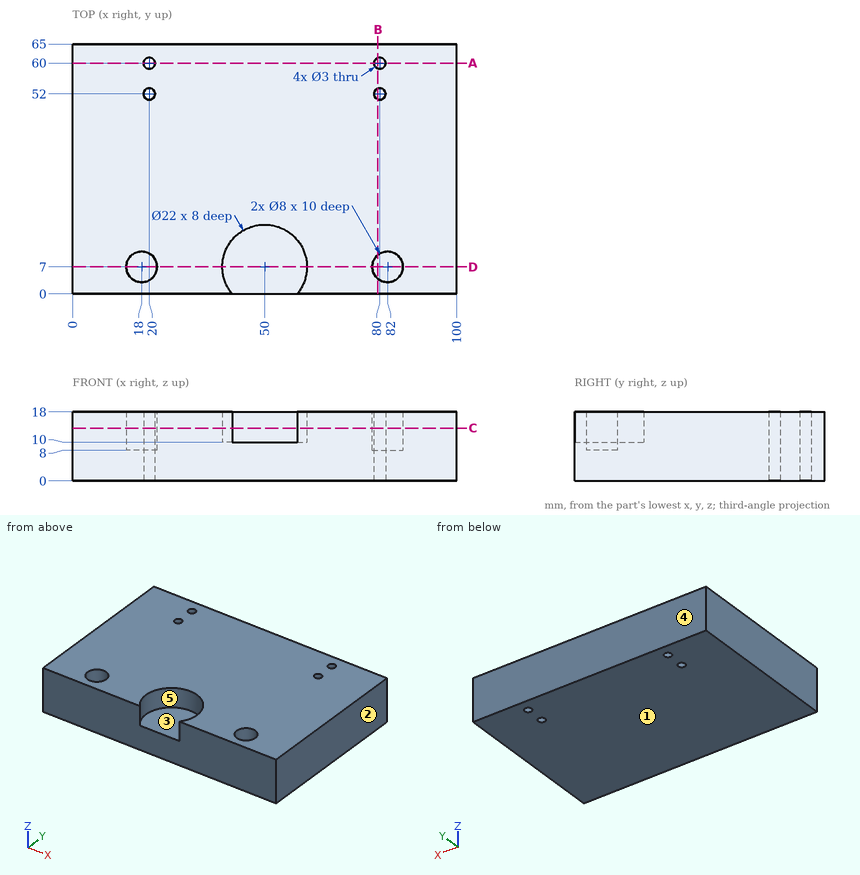
Part print with two shaded views. Sizes in mm from the minimum x, y, z corner. A direction names the side the tool comes from. Round coordinates to 2 decimals unless told otherwise and drop trailing zeros. Order: outer loops, then holes, each group sorted by start corner. A loop starts at its lowest first (then second) coordinate and runs counter-clockwise, first axis right, second up. Notation, with made-up numbers: (-33.5, 14.25) -> (1.5, 14.25) arc R16 cw to (1.5, 44.25) -> close; hole circle Ø2 at (8.25, 87). An arc over 180 degrees is marked (long way). Use one line per item in the form item = value.
Item 1: Drill centre lines: line 1 (Y direction, x = 20, z = 6.5); line 2 (Y direction, x = 82, z = 12.75); line 3 (X direction, y = 8, z = 13). Where is each one in solid material? Low to high.
Returned:
line_1 = 0 to 50.5, 53.5 to 58.5, 61.5 to 65
line_2 = 0 to 3, 11 to 65
line_3 = 0 to 14.13, 21.87 to 39.05, 60.95 to 78.13, 85.87 to 100
Item 2: Cut at B-B, the plane x = 79.5. Write the cut outline in (y, z), and give its area (3 significant figures).
Returned:
outline = (0, 0) -> (50.59, 0) -> (50.59, 18) -> (10.12, 18) -> (10.12, 8) -> (3.88, 8) -> (3.88, 18) -> (0, 18) -> close; (53.41, 0) -> (58.59, 0) -> (58.59, 18) -> (53.41, 18) -> close; (61.41, 0) -> (65, 0) -> (65, 18) -> (61.41, 18) -> close
area = 1,010 mm^2
Item 3: Cut at D-D, the plane y = 7. Write the cut outline in (x, z).
Returned:
outline = (0, 0) -> (100, 0) -> (100, 18) -> (86, 18) -> (86, 8) -> (78, 8) -> (78, 18) -> (61, 18) -> (61, 10) -> (39, 10) -> (39, 18) -> (22, 18) -> (22, 8) -> (14, 8) -> (14, 18) -> (0, 18) -> close
Item 4: Cut at A-A, the plane y = 60. Write the cut outline in (x, z), and give its area (3 significant figures).
Returned:
outline = (0, 0) -> (18.5, 0) -> (18.5, 18) -> (0, 18) -> close; (21.5, 0) -> (78.5, 0) -> (78.5, 18) -> (21.5, 18) -> close; (81.5, 0) -> (100, 0) -> (100, 18) -> (81.5, 18) -> close
area = 1,690 mm^2
Item 5: Tool access for the marked faces 4 and 5: list every direction of +Z, -Z, +X, -X, +Y, -Y with a clear straight run to the whole face (end or side of a thin tool).
Returned:
face_4 = +Z, -Z, +X, -X, +Y
face_5 = +Z
Item 6: Flat gauge pins, fed straight in: pin 1 Ø5.5 at (x, y) = (50.5, 8.5) entering from +Z; pin 2 Ø6.5 at (x, y) = (80.5, 6.5) entering from +Z; pin 3 Ø7 at (x, y) = (82, 7) entering from +Z. Where does each tip first touch, or does it go through?
Returned:
pin_1 = 10
pin_2 = 18
pin_3 = 8
Item 7: Pull direction X, two halves, no side cores. Call the marked faces 1, 2 and 3: released by +X, released by -X, zero draft, split by the parting line, or undercut.
Returned:
face_1 = zero draft
face_2 = released by +X
face_3 = undercut
Item 8: Cut at C-C, the plane z = 13.75. Write the cut outline in (x, y), and give its area (3 significant figures).
Returned:
outline = (0, 0) -> (41.51, 0) arc R11 cw (long way) to (58.49, 0) -> (100, 0) -> (100, 65) -> (0, 65) -> close; hole circle Ø8 at (18, 7); hole circle Ø3 at (20, 52); hole circle Ø3 at (20, 60); hole circle Ø8 at (82, 7); hole circle Ø3 at (80, 52); hole circle Ø3 at (80, 60)
area = 6,040 mm^2
